Read the model definition and answer for the solid it produces. Units are mm, in the model's axes. Face numbers are marked on the shaded views. A direction names the side the tool comes from. Coordinates: 2 decimals unless noted, no trailing zeros. Order: outer loops, then holes, each group sorted by start corner. A loop starts at its lowest first (then second) coordinate and runs counter-clockwise, first axis right, second up.
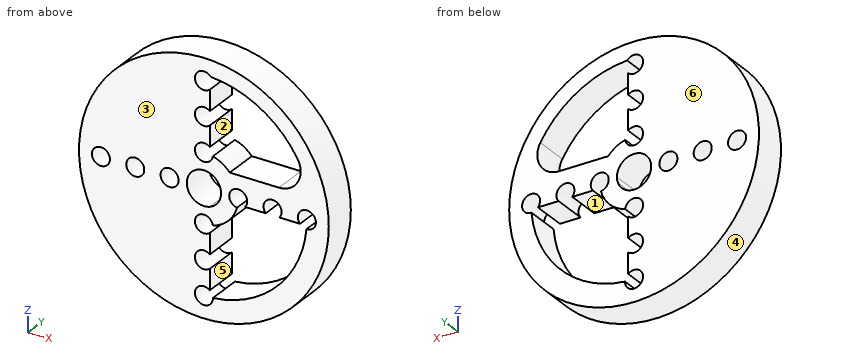
```python
from build123d import *

# Parameters (mm, degrees)
F0_R     = 29.105
F1_DEPTH = 8
F2_D     = 4.2
F2_DEPTH = 12.7
F2_TIP   = 1.2618073
F3_R     = 5.08


with BuildPart() as f1:
    # F0 (on Front) → F1 (new body)
    with BuildSketch(Plane.XZ):
        Circle(F0_R)
        with BuildLine():
            ThreePointArc((25.3854070023, 0), (18.4286183858, -17.4586629804), (1.3712233387, -25.3483458085))
            ThreePointArc((1.3712233387, -25.3483458085), (-25.3854070023, 0), (1.3712233387, 25.3483458085))
            ThreePointArc((1.3712233387, 25.3483458085), (16.5113444887, 19.2819706422), (24.8353761494, 5.255756862))
            ThreePointArc((24.8353761494, 5.255756862), (25.2475248319, 2.6422298411), (25.3854070023, 0))
        make_face(mode=Mode.SUBTRACT)
        with BuildLine():
            Line((1.3712233387, -23.9607960334), (1.3712233387, -15.9411337914))
            ThreePointArc((1.3712233387, -15.9411337914), (-16, 0), (1.3712233387, 15.9411337914))
            Line((1.3712233387, 15.9411337914), (1.3712233387, 23.9607960334))
            ThreePointArc((1.3712233387, 23.9607960334), (-24, 0), (1.3712233387, -23.9607960334))
        make_face()
        with BuildLine():
            Line((1.3712233387, -15.9411337914), (1.3712233387, -7.8816081199))
            ThreePointArc((1.3712233387, -7.8816081199), (-8, 0), (1.3712233387, 7.8816081199))
            Line((1.3712233387, 7.8816081199), (1.3712233387, 15.9411337914))
            ThreePointArc((1.3712233387, 15.9411337914), (-16, 0), (1.3712233387, -15.9411337914))
        make_face()
        with BuildLine():
            ThreePointArc((1.3712233387, -3.7576251217), (-3.2775671888, 2.2929355252), (4, 0))
            ThreePointArc((4, 0), (3.9389053429, -0.6964371472), (3.75748765, -1.3716))
            Line((3.75748765, -1.3716), (7.88154258, -1.3716))
            ThreePointArc((7.88154258, -1.3716), (7.970330628, -0.6883528747), (8, 0))
            ThreePointArc((8, 0), (7.4916851205, 2.8061814011), (6.031336486, 5.255756862))
            Line((6.031336486, 5.255756862), (1.3712233387, 5.255756862))
            Line((1.3712233387, 5.255756862), (1.3712233387, 7.8816081199))
            ThreePointArc((1.3712233387, 7.8816081199), (-8, 0), (1.3712233387, -7.8816081199))
            Line((1.3712233387, -7.8816081199), (1.3712233387, -3.7576251217))
        make_face()
        with BuildLine():
            Line((1.3712233387, -25.3483458085), (1.3712233387, -23.9607960334))
            ThreePointArc((1.3712233387, -23.9607960334), (-24, 0), (1.3712233387, 23.9607960334))
            Line((1.3712233387, 23.9607960334), (1.3712233387, 25.3483458085))
            ThreePointArc((1.3712233387, 25.3483458085), (-25.3854070023, 0), (1.3712233387, -25.3483458085))
        make_face()
        with BuildLine():
            ThreePointArc((23.960774475, -1.3716), (16.9704293601, -16.9706961358), (1.3712233387, -23.9607960334))
            Line((1.3712233387, -23.9607960334), (1.3712233387, -25.3483458085))
            ThreePointArc((1.3712233387, -25.3483458085), (18.4286183858, -17.4586629804), (25.3854070023, 0))
            ThreePointArc((25.3854070023, 0), (25.2475248319, 2.6422298411), (24.8353761494, 5.255756862))
            Line((24.8353761494, 5.255756862), (23.4174511808, 5.255756862))
            ThreePointArc((23.4174511808, 5.255756862), (23.8539182142, 2.6439716016), (24, 0))
            ThreePointArc((24, 0), (23.9901916145, -0.6860803892), (23.960774475, -1.3716))
        make_face()
        with BuildLine():
            ThreePointArc((8, 0), (7.970330628, -0.6883528747), (7.88154258, -1.3716))
            Line((7.88154258, -1.3716), (15.9411013873, -1.3716))
            ThreePointArc((15.9411013873, -1.3716), (15.9852685651, -0.686432008), (16, 0))
            ThreePointArc((16, 0), (15.7764756741, 2.6651107487), (15.1121480871, 5.255756862))
            Line((15.1121480871, 5.255756862), (6.031336486, 5.255756862))
            ThreePointArc((6.031336486, 5.255756862), (7.4916851205, 2.8061814011), (8, 0))
        make_face()
        with BuildLine():
            ThreePointArc((16, 0), (15.9852685651, -0.686432008), (15.9411013873, -1.3716))
            Line((15.9411013873, -1.3716), (23.960774475, -1.3716))
            ThreePointArc((23.960774475, -1.3716), (23.9901916145, -0.6860803892), (24, 0))
            ThreePointArc((24, 0), (23.8539182142, 2.6439716016), (23.4174511808, 5.255756862))
            Line((23.4174511808, 5.255756862), (15.1121480871, 5.255756862))
            ThreePointArc((15.1121480871, 5.255756862), (15.7764756741, 2.6651107487), (16, 0))
        make_face()
        with BuildLine():
            ThreePointArc((3.75748765, -1.3716), (2.828285359, -2.8285688834), (1.3712233387, -3.7576251217))
            Line((1.3712233387, -3.7576251217), (1.3712233387, -7.8816081199))
            ThreePointArc((1.3712233387, -7.8816081199), (5.656719077, -5.6569894187), (7.88154258, -1.3716))
            Line((7.88154258, -1.3716), (3.75748765, -1.3716))
        make_face()
        with BuildLine():
            ThreePointArc((6.031336486, 5.255756862), (3.9272441605, 6.9697025262), (1.3712233387, 7.8816081199))
            Line((1.3712233387, 7.8816081199), (1.3712233387, 5.255756862))
            Line((1.3712233387, 5.255756862), (6.031336486, 5.255756862))
        make_face()
    extrude(amount=-F1_DEPTH)

    # F2
    with Locations(Plane.XZ):
        with Locations((0, 24), (24, 0), (0, -24), (-24, 0), (0, 16), (16, 0), (0, -16), (-16, 0), (0, 8), (8, 0), (0, -8), (-8, 0)):
            Hole(F2_D / 2, depth=F2_DEPTH)
            with Locations((0, 0, -(F2_DEPTH + F2_TIP / 2))):  # 118° drill point
                Cone(0, F2_D / 2, F2_TIP, mode=Mode.SUBTRACT)

    # F3
    f3_edges = [f1.edges().sort_by_distance(p)[0] for p in [
        (24.835376, 4, 5.255757),
    ]]
    fillet(f3_edges, radius=F3_R)


solid = f1.part
```
1) A cutting plane is placed at C-C, the plane z = -12.5. Determine the outline of the cut face in (x, y).
A:
outline: (-26.28, 0) - (1.37, 0) - (1.37, 8) - (-26.28, 8) - close; (20.49, 0) - (26.28, 0) - (26.28, 8) - (20.49, 8) - close
2) Flat-ended cylindrical pins translate along their axes: pin 1 Ø2.5 at (x, y) = (14.5, 5.5) entering from +Z; pin 2 Ø3.5 at (x, z) = (0, 16) entering from -Y; pin 3 Ø4 at (y, z) = (4.5, 13) entering from +X; pin 4 Ø4 at (x, y) = (20, 3.5) entering from -Z. Find the tip coordinate at first contact, or state that the pin passes through.
A:
pin 1: stops at z = 25.91
pin 2: passes through
pin 3: stops at x = 26.95
pin 4: stops at z = -22.87
3) A cutting plane is placed at D-D, the plane x = 16. Determine the outline of the cut face in (y, z).
A:
outline: (0, -24.31) - (8, -24.31) - (8, -17.89) - (0, -17.89) - close; (0, 2.1) - (8, 2.1) - (8, 5.26) - (0, 5.26) - close; (0, 19.71) - (8, 19.71) - (8, 24.31) - (0, 24.31) - close
4) A cutting plane is placed at B-B, the plane y = 7.25. Determine the outline of the cut face in (x, z) (3 decimals), and give its area (3 significant figures).
A:
outline: circle Ø58.21 at (0, 0); hole circle Ø4.2 at (-24, 0); hole circle Ø4.2 at (-16, 0); hole circle Ø4.2 at (-8, 0); hole circle Ø8 at (0, 0); hole (1.371, -22.409) arc R2.1 ccw (long way) to (2.098, -23.908) arc R24 ccw to (23.908, -2.098) arc R2.1 ccw (long way) to (22.41, -1.372) - (17.59, -1.372) arc R2.1 ccw (long way) to (14.41, -1.372) - (9.59, -1.372) arc R2.1 ccw (long way) to (7.724, -2.082) arc R8 cw to (2.082, -7.724) arc R2.1 ccw (long way) to (1.371, -9.591) - (1.371, -14.409) arc R2.1 ccw (long way) to (1.371, -17.591) - close; hole (1.371, 9.591) arc R2.1 ccw (long way) to (2.082, 7.724) arc R8 cw to (6.031, 5.256) - (17.478, 5.256) arc R5.08 ccw to (21.851, 12.922) arc R25.385 ccw to (1.622, 25.334) arc R2.1 ccw (long way) to (1.371, 22.409) - (1.371, 17.591) arc R2.1 ccw (long way) to (1.371, 14.409) - close
area: 1,770 mm2
5) Determine the mould class of the marked faces 1, 2, 3 and 4 for opening direction X: pulls with the +X half, pulls with the -X half, needs draft (parallel to the pull), parting line crosses it, or undercut.
A:
face 1: undercut
face 2: undercut
face 3: needs draft
face 4: parting line crosses it
6) Which of the six approach directions +Z, -Z, +X, -X, +Y, -Y give full straight-line access (tool end or side, diameter ignored) to the marked faces 5 and 6?
A:
face 5: +Y, -Y
face 6: +Z, -Z, +X, -X, +Y
7) A cutting plane is placed at A-A, the plane x = 0. State how many separate pieces and enclosed holes the cut face has, and give its area (3 significant figures).
A:
separate pieces: 8
enclosed holes: 0
area: 200 mm2
8) Straight lines are drawn through the part: line 1 (Z direction, x = 15, y = 6.25) (3 decimals); line 2 (Z direction, x = 9, y = 2.25); line 3 (X direction, y = 3.5, z = -11.5). For each, find the intervals that lie inside material, in ascending order.
A:
line 1: z = -24.942 to -18.735, 1.847 to 5.256, 20.48 to 24.942
line 2: z = -27.68 to -22.25, 1.85 to 5.26, 23.74 to 27.68
line 3: x = -26.74 to 1.37, 21.07 to 26.74
